from build123d import *

# Parameters (mm, degrees)
F0_W           = 50
F0_H           = 50
F1_DEPTH       = 50
F3_D           = 2
F3_CBORE_D     = 10
F3_CBORE_DEPTH = 4
F4_W           = 25
F4_H           = 25
F5_DEPTH       = 25
F6_R           = 5


with BuildPart() as f1:
    # F0 (on Top) → F1 (new body)
    with BuildSketch(Plane.XY):
        Rectangle(F0_W, F0_H)
    extrude(amount=F1_DEPTH)

    # F3 (through all)
    with Locations(Plane.YZ.offset(25)):
        with Locations((15, 40)):
            CounterBoreHole(F3_D / 2, F3_CBORE_D / 2, F3_CBORE_DEPTH)

    # F4 (on face) → F5 (cut)
    with BuildSketch(Plane.XZ.offset(25)):
        with Locations((-12.5, 37.5)):
            Rectangle(F4_W, F4_H)
    extrude(amount=-F5_DEPTH, mode=Mode.SUBTRACT)

    # F6
    f6_edges = [f1.edges().sort_by_distance(p)[0] for p in [
        (-12.5, 0, 25),
        (-25, 0, 37.5),
        (0, 0, 37.5),
        (0, -12.5, 50),
        (0, -25, 37.5),
        (-12.5, -25, 25),
        (0, -12.5, 25),
        (-25, 12.5, 50),
        (12.5, -25, 50),
        (-25, -25, 12.5),
        (-12.5, 0, 50),
        (-25, -12.5, 25),
    ]]
    fillet(f6_edges, radius=F6_R)


solid = f1.part
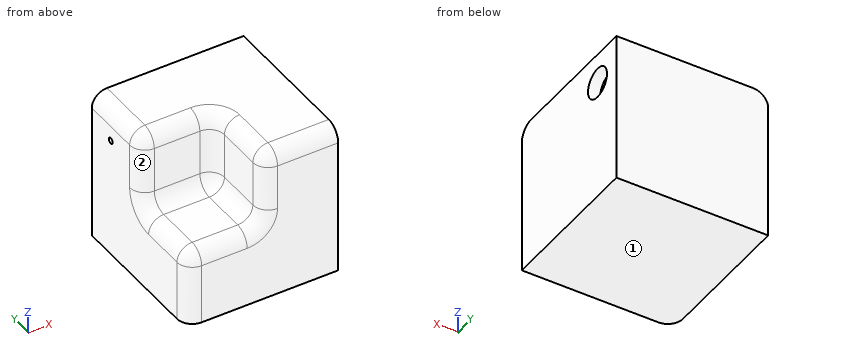
Could you check a few things on this model? Use its own coordinates, in mm. Face numbers are marked on the shaded views. A direction names the side the tool comes from. Give positions to 0.01 mm unless a question says otherwise; leave off trailing zeros. Order: outer loops, then holes, each group sorted by start corner. A loop starts at its lowest first (then second) coordinate and runs counter-clockwise, first axis right, second up. Notation, with made-up numbers: (-13.5, 26) - (42.5, 26) arc R21 ccw to (42.5, 63) - close; hole circle Ø1 at (-21, 20). An arc over 180 degrees is marked (long way). Return JSON: item names as keys, results as strings. Group by question number.
Q1. Will these pins go through, and if not, where does the flat tip stop? pin 1 Ø12 at (x, y) = (-9.5, -15.5) entering from +Z; pin 2 Ø7.5 at (y, z) = (-15, 37.5) entering from -X; pin 3 Ø7.5 at (x, z) = (-13, 34) entering from -Y.
Q2. Suppose I cut it at B-B, the plane y = 15. Please give me the cut outline in (x, z).
Q3. Suppose I cut it at D-D, the plane y = -10.5. Please give me the cut outline in (x, z), and give its area (3 significant figures).
Q4. Suppose I cut it at C-C, the plane x = -17. Please give me the cut outline in (y, z), and give its area (3 significant figures).
Q5. Suppose I cut it at A-A, the plane z = 40. Please give me the cut outline in (x, y), and give its area (3 significant figures).
Q6. Which directions (+Z, -Z, +X, -X, +Y, -Y) give clear straight access to the entire face, cutting with the end or side of a thin tool? Please do the marked faces 1 and 2.
Q7. Please list where these lines run through material, in increasing order: line 1 along Z through (x, y) = (4, 15); line 2 along Z through (x, y) = (24.1, 15); line 3 along Y through (x, z) = (2.5, 24). Write a range as [from, to].
Resolved:
{
 "1": {"pin 1": "stops at z = 25.23", "pin 2": "stops at x = 0", "pin 3": "stops at y = 0"},
 "2": {"outline": "(-25, 0) - (25, 0) - (25, 35) - (21, 35) - (21, 39) - (-25, 39) - close; (-25, 41) - (21, 41) - (21, 45) - (25, 45) - (25, 50) - (-20, 50) arc R5 ccw to (-25, 45) - close"},
 "3": {"outline": "(-25, 0) - (25, 0) - (25, 50) - (5, 50) arc R5 ccw to (0, 45) - (0, 30) arc R5 cw to (-5, 25) - (-20, 25) arc R5 ccw to (-25, 20) - close", "area": "1,870 mm2"},
 "4": {"outline": "(-25, 0) - (25, 0) - (25, 50) - (5, 50) arc R5 ccw to (0, 45) - (0, 30) arc R5 cw to (-5, 25) - (-20, 25) arc R5 ccw to (-25, 20) - close; hole circle Ø2 at (15, 40)", "area": "1,870 mm2"},
 "5": {"outline": "(-25, 5) arc R5 ccw to (-20, 0) - (-5, 0) arc R5 cw to (0, -5) - (0, -20) arc R5 ccw to (5, -25) - (25, -25) - (25, 10) - (21, 10) - (21, 14) - (-25, 14) - close; (-25, 16) - (21, 16) - (21, 20) - (25, 20) - (25, 25) - (-25, 25) - close", "area": "1,740 mm2"},
 "6": {"face 1": "-Z, +X, -X, +Y, -Y", "face 2": "+Z, -X, -Y"},
 "7": {"line 1": "z = [0, 39], [41, 50]", "line 2": "z = [0, 35], [45, 50]", "line 3": "y = [-24.98, 25]"}
}
